Could you check a few things on this model? Use its own coordinates, in mm. A direction names the side the tool comes from. Coordinates: 2 decimals unless noted, no trailing zeros. Write each loop counter-clockwise with the first axis right and the second up, starting at its lowest first coordinate (ties: lowest second). Pieces come first, ordered by that corner, then holes. Notation, with made-up numbers: (52.25, 56.25) - (101.25, 56.25) arc R24 cw to (101.25, 73.25) - close; hole circle Ø8 at (71, -33). An arc over 180 degrees is marked (long way). Answer as a JSON object with one key per item and string values. Group by question number.
1) On a 3-axis mill with a long thin cutter (end or side, diameter ignored), from which of +Z, -Z, +X, -X, +Y, -Y can I reach the whole of each face in a straight line? I mean faces 1 (the flat face through (-26, 4, 0)), 2 (the flat face through (-27.352, 5, 22)), 3 (the cylindrical face through (-23.353, 5.287, 2.465)), 4 (the flat face through (-22.352, 5, 22)). Say none if no direction works.
2) Please list where these lines run through material, in increasing order: line 1 along X through (y, z) = (6.2, 29); line 2 along Z through (x, y) = (-19.5, 5.15); line 3 along Z through (x, y) = (-24, 6.3).
3) If we section it at A-A (y = 6.05): Write out the boundary of the cut face in (x, z).
4) Will this pin go through, and if not, where does the flat tip stop? pin 1 Ø2.5 at (y, z) = (5, 20.5) entering from +X.
5) If we section it at C-C (z = 32): Write out the boundary of the cut face in (x, y), plus the area to 3 significant figures.
6) If we section it at B-B (x = -24): Write out the boundary of the cut face in (y, z).
7) We'd pull the mould along Y, two halves only. Please class faces 5 (the flat face through (-25, 7.721, 41)), 6 (the flat face through (-25, 5, 5)), 7 (the flat face through (-33, 5, 45)): released by +Y, released by -Y, zero draft, split by the parting line, or undercut.
8) If we section it at D-D (x = -20.5): Write out the boundary of the cut face in (y, z).
```python
from build123d import *

# Parameters (mm, degrees)
SKETCH1_W           = 5
SKETCH1_H           = 5
BOSS_EXTRUDE1_DEPTH = 45
SKETCH2_W           = 26
SKETCH2_H           = 5
BOSS_EXTRUDE2_DEPTH = 15
SKETCH3_R           = 1.5
CUT_EXTRUDE1_DEPTH  = 5


with BuildPart() as part:
    # Sketch1 → Boss-Extrude1 (new body)
    with BuildSketch(Plane.XY):
        with Locations((-24.851797929, 5.221320947)):
            Rectangle(SKETCH1_W, SKETCH1_H)
    extrude(amount=BOSS_EXTRUDE1_DEPTH)

    # Sketch2 → Boss-Extrude2 (add)
    with BuildSketch(Plane.XY.offset(45)):
        with Locations((-24.851797929, 5.221320947)):
            Rectangle(SKETCH2_W, SKETCH2_H)
    extrude(amount=BOSS_EXTRUDE2_DEPTH)

    # Sketch3 → Cut-Extrude1 (cut)
    with BuildSketch(Plane(origin=(0, 0, 0), x_dir=(-1, 0, 0), z_dir=(0, 0, -1))):
        with Locations((24.851797929, 5.221320947)):
            Circle(SKETCH3_R)
    extrude(amount=-CUT_EXTRUDE1_DEPTH, mode=Mode.SUBTRACT)


solid = part.part
```
Here are the results:
{
 "1": {"face 1": "-Z, +X, -X, +Y, -Y", "face 2": "-Z, -X, +Y, -Y", "face 3": "-Z", "face 4": "-Z, +X, +Y, -Y"},
 "2": {"line 1": "x = -27.35 to -22.35", "line 2": "z = 45 to 60", "line 3": "z = 5 to 60"},
 "3": {"outline": "(-37.85, 45) - (-27.35, 45) - (-27.35, 0) - (-26.1, 0) - (-26.1, 5) - (-23.6, 5) - (-23.6, 0) - (-22.35, 0) - (-22.35, 45) - (-11.85, 45) - (-11.85, 60) - (-37.85, 60) - close"},
 "4": {"pin 1": "stops at x = -22.35"},
 "5": {"outline": "(-27.35, 2.72) - (-22.35, 2.72) - (-22.35, 7.72) - (-27.35, 7.72) - close", "area": "25.0 mm²"},
 "6": {"outline": "(2.72, 0) - (3.99, 0) - (3.99, 5) - (6.46, 5) - (6.46, 0) - (7.72, 0) - (7.72, 60) - (2.72, 60) - close"},
 "7": {"face 5": "released by +Y", "face 6": "undercut", "face 7": "zero draft"},
 "8": {"outline": "(2.72, 45) - (7.72, 45) - (7.72, 60) - (2.72, 60) - close"}
}
